Could you check a few things on this drawing? It's one solid part, dimensions in mm from its lowest x, y, z. A direction names the side the tool comes from. Coordinates: 2 decimals unless noted, no trailing zeros. Order: outer loops, then holes, each group sorted by start corner. A loop starts at its lowest first (then second) coordinate and runs counter-clockwise, first axis right, second up.
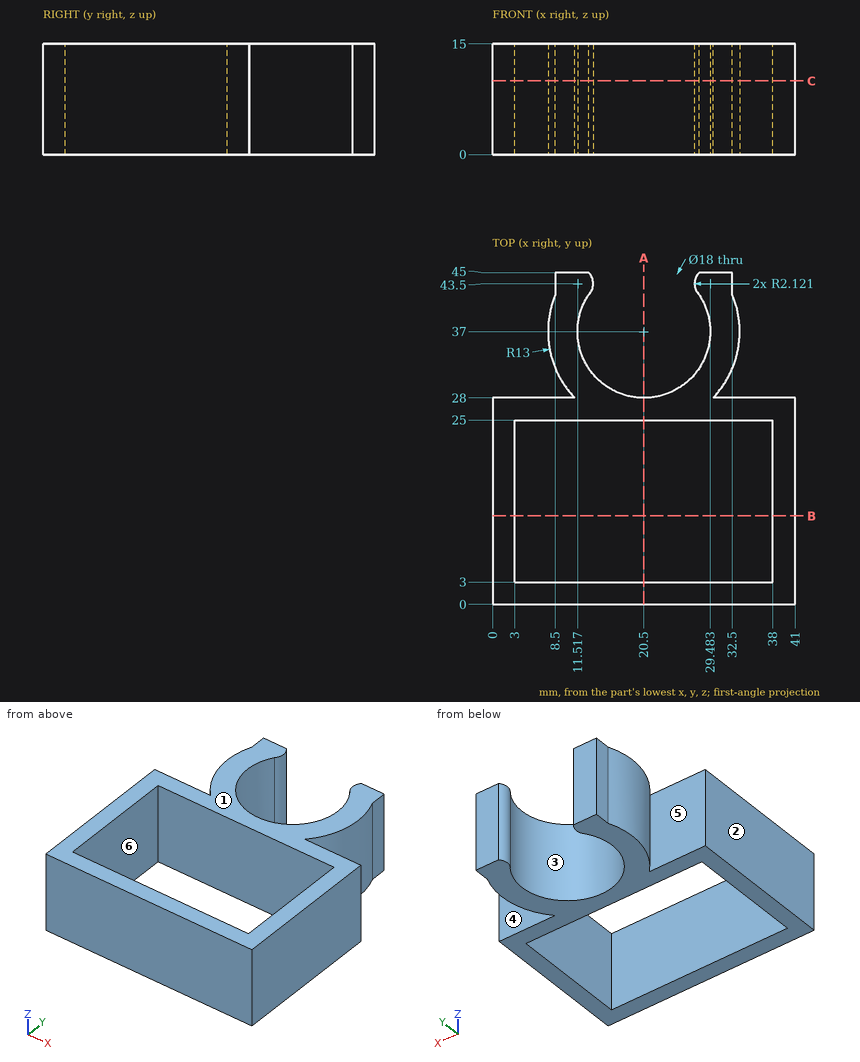
Q1. I need wall thicknesses on L1, parallel to X at y = 8.5, z = 2; L2, parallel to X at y = 37, z = 7.5; L3, parallel to Y at x = 4, z = 1. Which ranges of each line are inside material? Lowest first, please.
Q2. Will these pins go through, and if not, where does the flat tip stop? pin 1 (7.5 mm diameter, centred on y = 10, z = 9, fed in from -X); pin 2 (3.5 mm diameter, centred on y = 43, z = 7.5, fed in from +X) (1 decimal); pin 3 (11 mm diameter, centred on x = 20.5, y = 37, fed in from +Z); pin 4 (3.5 mm diameter, centred on x = 3.5, z = 8.5, fed in from +Y).
Q3. We'd pull the mould along X, two halves only. Please class the marked faces 1, 2 and 3: pulls with the +X half, pulls with the -X half, needs draft (parallel to the pull), parting line crosses it, or undercut.
Q4. If we section it at C-C on z = 10: Write out the boundary of the cut face in (x, y).
Q5. If we section it at A-A on x = 20.5: Write out the boundary of the cut face in (y, z), then the cut area to 3 significant figures.
Q6. If we section it at B-B on y = 12: Write out the boundary of the cut face in (x, z), then the cut area to 3 significant figures.
Q7. For the marked faces 4, 5 and 6, which set-ups out of +Z, -Z, +X, -X, +Y, -Y let a thin tool reach every point of the face, with its end or its side?
Reply:
1. L1: x = 0 to 3, 38 to 41
1. L2: x = 7.5 to 11.5, 29.5 to 33.5
1. L3: y = 0 to 3, 25 to 28
2. pin 1: stops at x = 0
2. pin 2: stops at x = 32.8
2. pin 3: passes through
2. pin 4: stops at y = 28
3. face 1: needs draft
3. face 2: pulls with the -X half
3. face 3: undercut
4. outline: (0, 0) - (41, 0) - (41, 28) - (29.88, 28) arc R13 ccw to (32.5, 42) - (32.5, 45) - (27.98, 45) arc R2.12 ccw to (27.98, 42) arc R9 cw (long way) to (13.02, 42) arc R2.12 ccw to (13.02, 45) - (8.5, 45) - (8.5, 42) arc R13 ccw to (11.12, 28) - (0, 28) - close; hole (3, 3) - (38, 3) - (38, 25) - (3, 25) - close
5. outline: (0, 0) - (3, 0) - (3, 15) - (0, 15) - close; (25, 0) - (28, 0) - (28, 15) - (25, 15) - close
5. area: 90.0 mm2
6. outline: (0, 0) - (3, 0) - (3, 15) - (0, 15) - close; (38, 0) - (41, 0) - (41, 15) - (38, 15) - close
6. area: 90.0 mm2
7. face 4: +Z, -Z, +X
7. face 5: +Z, -Z, -X
7. face 6: +Z, -Z
